Here's how the part is built. I have some questions about the finished solid (model axes, mm). Round coordinates to 2 decimals unless told otherwise and drop trailing zeros. Loops run counter-clockwise (first coordinate to the right, second up) from the corner with the lowest first, then second, coordinate; pieces in that order, holes last. Notation, with made-up numbers: (21, 66) -> (32, 66) arc R26 cw to (32, 88) -> close; hole circle Ø2 at (43.5, -13.5). An arc over 180 degrees is marked (long way). Use CSV: the item, a comma, the result in double quotes. Start each with the question number.
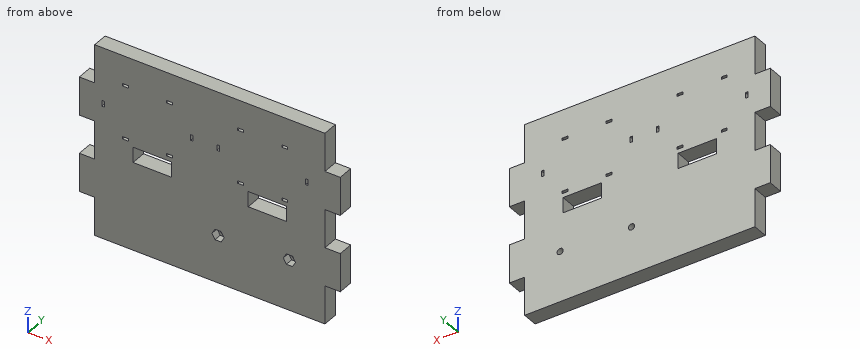
from build123d import *

# Parameters (mm, degrees)
SKETCH1_W           = 120
SKETCH1_H           = 100
SKETCH1_R           = 1.6
SKETCH1_W_2         = 3
SKETCH1_H_2         = 1.3
SKETCH1_W_3         = 1.3
SKETCH1_H_3         = 3
BOSS_EXTRUDE1_DEPTH = 8
CUT_EXTRUDE1_DEPTH  = 4
SKETCH3_W           = 20
SKETCH3_H           = 8
BOSS_EXTRUDE2_DEPTH = 8
CUT_EXTRUDE3_REACH  = 86.782
SKETCH5_W           = 20
SKETCH5_H           = 8


with BuildPart() as part:
    # Sketch1 → Boss-Extrude1 (new body)
    with BuildSketch(Plane(origin=(0, 0, 0), x_dir=(1, 0, 0), z_dir=(0, 1, 0))):
        Rectangle(SKETCH1_W, SKETCH1_H)
        with Locations(Location((41.5, 23.7, 0), (0, 0, 270))):
            Circle(SKETCH1_R, mode=Mode.SUBTRACT)
        with Locations(Location((4.3, 25.2, 0), (0, 0, 270))):
            Circle(SKETCH1_R, mode=Mode.SUBTRACT)
        with Locations((39, -6.85)):
            Rectangle(SKETCH1_W_2, SKETCH1_H_2, mode=Mode.SUBTRACT)
        with Locations((16, -6.85)):
            Rectangle(SKETCH1_W_2, SKETCH1_H_2, mode=Mode.SUBTRACT)
        with Locations((4.35, -20.75)):
            Rectangle(SKETCH1_W_3, SKETCH1_H_3, mode=Mode.SUBTRACT)
        with Locations((50.65, -20.75)):
            Rectangle(SKETCH1_W_3, SKETCH1_H_3, mode=Mode.SUBTRACT)
        with Locations((39, -34.65)):
            Rectangle(SKETCH1_W_2, SKETCH1_H_2, mode=Mode.SUBTRACT)
        with Locations((16, -34.65)):
            Rectangle(SKETCH1_W_2, SKETCH1_H_2, mode=Mode.SUBTRACT)
        with Locations((-21, -34.65)):
            Rectangle(SKETCH1_W_2, SKETCH1_H_2, mode=Mode.SUBTRACT)
        with Locations((-44, -34.65)):
            Rectangle(SKETCH1_W_2, SKETCH1_H_2, mode=Mode.SUBTRACT)
        with Locations((-55.65, -20.75)):
            Rectangle(SKETCH1_W_3, SKETCH1_H_3, mode=Mode.SUBTRACT)
        with Locations((-44, -6.85)):
            Rectangle(SKETCH1_W_2, SKETCH1_H_2, mode=Mode.SUBTRACT)
        with Locations((-9.35, -20.75)):
            Rectangle(SKETCH1_W_3, SKETCH1_H_3, mode=Mode.SUBTRACT)
        with Locations((-21, -6.85)):
            Rectangle(SKETCH1_W_2, SKETCH1_H_2, mode=Mode.SUBTRACT)
    extrude(amount=BOSS_EXTRUDE1_DEPTH)

    # Sketch2 → Cut-Extrude1 (cut)
    with BuildSketch(Plane(origin=(0, 0, 0), x_dir=(-1, 0, 0), z_dir=(0, -1, 0))):
        Polygon((-7.475426481, 25.2), (-5.88771324, 22.45), (-2.71228676, 22.45), (-1.124573519, 25.2), (-2.71228676, 27.95), (-5.88771324, 27.95), align=None)
        Polygon((-44.675426481, 23.7), (-43.08771324, 20.95), (-39.91228676, 20.95), (-38.324573519, 23.7), (-39.91228676, 26.45), (-43.08771324, 26.45), align=None)
    extrude(amount=-CUT_EXTRUDE1_DEPTH, mode=Mode.SUBTRACT)

    # Sketch3 → Boss-Extrude2 (add)
    with BuildSketch(Plane.ZY.offset(60)):
        with Locations((-20, 4)):
            Rectangle(SKETCH3_W, SKETCH3_H)
        with Locations((20, 4)):
            Rectangle(SKETCH3_W, SKETCH3_H)
    boss_extrude2 = extrude(amount=BOSS_EXTRUDE2_DEPTH)

    # Mirror1: Boss-Extrude2 across plane
    add(boss_extrude2.mirror(Plane.ZY))

    # Sketch5 → Cut-Extrude3 (cut, up to next)
    with BuildSketch(Plane(origin=(0, 0, 0), x_dir=(-1, 0, 0), z_dir=(0, -1, 0)), mode=Mode.PRIVATE) as cut_extrude3_sk1:
        with Locations((30, 0)):
            Rectangle(SKETCH5_W, SKETCH5_H)
    cut_extrude3_tool1 = extrude(cut_extrude3_sk1.sketch, amount=-CUT_EXTRUDE3_REACH, mode=Mode.PRIVATE) & part.part
    cut_extrude3 = cut_extrude3_tool1.solids().sort_by_distance((-30, 0, 0))[0]
    add(cut_extrude3, mode=Mode.SUBTRACT)

    # Mirror2: Cut-Extrude3 across plane
    add(cut_extrude3.mirror(Plane.ZY), mode=Mode.SUBTRACT)


solid = part.part
Q1. I need wall thicknesses on line 1 along Z through (x, y) = (27, 7.25); line 2 along Z through (x, y) = (4.3, 6.1); line 3 along Z through (x, y) = (41.5, 6.75). Which ranges of each line are inside material? Lowest first, please.
Q2. I want a section at A-A, the plane y = 2.5. Count the separate pieces of the cut face and the enclosed holes in it, then the cut area to 3 significant figures.
Q3. I want a section at B-B, the plane z = -42. List the corners of the cut face in (x, y) for me.
Q4. Will these pins go through, and if not, where does the flat tip stop? pin 1 Ø2 at (y, z) = (3, 38) entering from +X; pin 2 Ø1.4 at (y, z) = (5, 6.5) entering from -X; pin 3 Ø1.9 at (x, z) = (41.5, -23.7) entering from -Y.
Values found:
1,line 1,"-50 to -4, 4 to 50"
1,line 2,"-50 to -26.8, -23.6 to 19.25, 22.25 to 50"
1,line 3,"-50 to -25.3, -22.1 to 50"
2,separate pieces,"1"
2,enclosed holes,"16"
2,area,"12,200 mm2"
3,outline,"(-60, 0) -> (60, 0) -> (60, 8) -> (-60, 8) -> close"
4,pin 1,"x = 60"
4,pin 2,"x = -60"
4,pin 3,"through"
